The model under review builds one solid part; all positions refer to its coordinate system, in mm. Face numbers are marked on the shaded views. A direction names the side the tool comes from. Coordinates: 2 decimals unless noted, no trailing zeros. Write each loop counter-clockwise with the first axis right and the second up, starting at its lowest first coordinate (ties: lowest second). Pieces come first, ordered by that corner, then holes. Notation, with made-up numbers: (34.5, -28.75) - (46.5, -28.75) arc R10 cw to (46.5, -16.75) - close; hole circle Ø7 at (-24, -16). An arc over 180 degrees is marked (long way). Return JSON: item names as keys, results as strings. Group by question number.
(1) To check wall thickness, follow L1, parallel to X at y = -32, z = -29; L2, parallel to Z at x = -15, y = -6.5; L3, parallel to X at y = -39, z = -33.5. State the ranges of each line that lie inside material, in increasing order. Write a range as from..to.
(2) For pin 1 Ø3 at (x, y) = (18, -31.5) entering from +Z; pin 2 Ø12 at (x, y) = (-13, -12) entering from -Z; pin 3 Ø6 at (x, z) = (-10.5, -13.5) entering from +Y; pin 4 Ø1 at (y, z) = (-37.5, -35.5) entering from +X, all flat-tipped, find the tip position at first contact; note any pin that passes through.
(3) We need section C-C on z = -40. State the section outline as (x, y) points, then the cut area to 3 significant figures.
(4) We need section B-B on y = -6. State the section outline as (x, z) points.
(5) We need section D-D on x = 4.5. State the section outline as (y, z) points, then the cut area to 3 significant figures.
(6) Tool access review of the marked faces 1 and 2: name each direction out of +Z, -Z, +X, -X, +Y, -Y from which nothing blocks a thin tool from reaching the whole face with its end or side.
(7) We need section A-A on y = -21. State the section outline as (x, z) points, then the cut area to 3 significant figures.
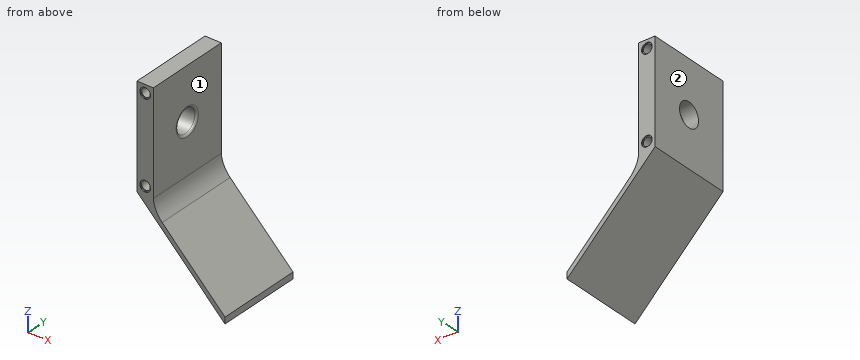
```python
from build123d import *

# Parameters (mm, degrees)
SKETCH1_W           = 25
SKETCH1_H           = 50
SKETCH1_R           = 3.4
BOSS_EXTRUDE1_DEPTH = 3
SKETCH2_W           = 50
SKETCH2_H           = 3
BOSS_EXTRUDE2_DEPTH = 8
SKETCH3_W           = 8
SKETCH3_H           = 50
BOSS_EXTRUDE3_DEPTH = 42
SKETCH4_R           = 2.65
CUT_EXTRUDE1_DEPTH  = 0.5
SKETCH5_R           = 5.888972746
CUT_EXTRUDE2_DEPTH  = 9
FILLET2_R           = 1
SKETCH6_R           = 12.6
BOSS_EXTRUDE4_DEPTH = 2
FILLET4_R           = 1
SKETCH8_R           = 1.589780168
SKETCH8_R_2         = 1.777428262
CUT_EXTRUDE3_DEPTH  = 10
SKETCH9_W           = 49.021678163
SKETCH9_H           = 20.976854622
CUT_EXTRUDE4_DEPTH  = 68.79439129
SKETCH11_R          = 2.1
CUT_EXTRUDE5_DEPTH  = 59.480168703
SKETCH14_R          = 2.6
CUT_EXTRUDE6_DEPTH  = 0.5
BOSS_EXTRUDE5_DEPTH = 42
FILLET5_R           = 15


with BuildPart() as part:
    # Sketch1 → Boss-Extrude1 (new body)
    with BuildSketch(Plane(origin=(0, 0, 0), x_dir=(1, 0, 0), z_dir=(0, 1, 0))):
        with Locations((2.276951673, 11.384758364)):
            Rectangle(SKETCH1_W, SKETCH1_H)
        with Locations(Location((1.276951673, 11.384758364, 0), (0, 0, 270))):
            Circle(SKETCH1_R, mode=Mode.SUBTRACT)
    extrude(amount=BOSS_EXTRUDE1_DEPTH)

    # Sketch2 → Boss-Extrude2 (add)
    with BuildSketch(Plane.ZY.offset(10.223048327)):
        with Locations((-11.384758364, 1.5)):
            Rectangle(SKETCH2_W, SKETCH2_H)
    extrude(amount=BOSS_EXTRUDE2_DEPTH)

    # Sketch3 → Boss-Extrude3 (add)
    with BuildSketch(Plane.XZ):
        with Locations((-14.223048327, -11.384758364)):
            Rectangle(SKETCH3_W, SKETCH3_H)
    extrude(amount=BOSS_EXTRUDE3_DEPTH)

    # Sketch4 → Cut-Extrude1 (cut)
    with BuildSketch(Plane(origin=(0, 3, 0), x_dir=(1, 0, 0), z_dir=(0, 1, 0))):
        with Locations(Location((-14.223048327, 32.384758364, 0), (0, 0, 270))):
            Circle(SKETCH4_R)
        with Locations(Location((-14.223048327, -9.615241636, 0), (0, 0, 270))):
            Circle(SKETCH4_R)
    cut_extrude1 = extrude(amount=-CUT_EXTRUDE1_DEPTH, mode=Mode.SUBTRACT)

    # Mirror1: Cut-Extrude1 across plane
    add(cut_extrude1.mirror(Plane.ZX.offset(-19.5)), mode=Mode.SUBTRACT)

    # Sketch5 → Cut-Extrude2 (cut)
    with BuildSketch(Plane.ZY.offset(18.223048327)):
        with Locations((-11.836279124, -21)):
            Circle(SKETCH5_R)
    extrude(amount=-CUT_EXTRUDE2_DEPTH, mode=Mode.SUBTRACT)

    # Fillet2
    fillet2_edges = [part.edges().sort_by_distance(p)[0] for p in [
        (-10.223048327, -21, -17.72525187),
    ]]
    fillet(fillet2_edges, radius=FILLET2_R)

    # Mirror2: Cut-Extrude1 across plane
    add(cut_extrude1.mirror(Plane.ZY.offset(1.723048327)), mode=Mode.SUBTRACT)

    # Sketch6 → Boss-Extrude4 (add)
    with BuildSketch(Plane(origin=(0, 3, 0), x_dir=(1, 0, 0), z_dir=(0, 1, 0))):
        with BuildLine():
            Line((14.776951673, 5.825082115), (14.776951673, 16.944434614))
            ThreePointArc((14.776951673, 16.944434614), (-13.323048327, 11.384758364), (14.776951673, 5.825082115))
        make_face()
        with Locations(Location((1.276951673, 11.384758364, 0), (0, 0, 270))):
            Circle(SKETCH6_R, mode=Mode.SUBTRACT)
    extrude(amount=BOSS_EXTRUDE4_DEPTH)

    # Fillet4
    # the kernel refuses this fillet: 1 mm, written as the material it takes off along each edge
    with BuildSketch(Plane(origin=(14.776951673, 5, -3.325082115), x_dir=(0, -1, 0), z_dir=(0, 0, -1))) as fillet4_piece_1:
        with BuildLine():
            CenterArc((FILLET4_R, FILLET4_R), FILLET4_R, 180, 90)
            Line((0, FILLET4_R), (0, 0))
            Line((0, 0), (FILLET4_R, 0))
        make_face()
    extrude(amount=16.119352499, mode=Mode.SUBTRACT)

    # Sketch8 → Cut-Extrude3 (cut)
    with BuildSketch(Plane(origin=(0, 3, 0), x_dir=(1, 0, 0), z_dir=(0, 1, 0))):
        with Locations(Location((1.276951673, 19.884758364, 0), (0, 0, 270))):
            Circle(SKETCH8_R)
        with Locations(Location((1.276951673, 2.884758364, 0), (0, 0, 270))):
            Circle(SKETCH8_R_2)
    extrude(amount=-CUT_EXTRUDE3_DEPTH, mode=Mode.SUBTRACT)

    # Sketch9 → Cut-Extrude4 (cut, through all)
    with BuildSketch(Plane.XY.offset(13.615241636)):
        with Locations((-9.733887409, 10.488427311)):
            Rectangle(SKETCH9_W, SKETCH9_H)
    extrude(amount=-CUT_EXTRUDE4_DEPTH, mode=Mode.SUBTRACT)

    # Sketch11 → Cut-Extrude5 (cut, through all)
    with BuildSketch(Plane(origin=(0, 0, 0), x_dir=(1, 0, 0), z_dir=(0, 1, 0))):
        with Locations(Location((-14.223048327, 32.384758364, 0), (0, 0, 270))):
            Circle(SKETCH11_R)
    cut_extrude5 = extrude(amount=-CUT_EXTRUDE5_DEPTH, mode=Mode.SUBTRACT)

    # Mirror3: Cut-Extrude5 across plane
    add(cut_extrude5.mirror(Plane.XY.offset(-11.384758364)), mode=Mode.SUBTRACT)

    # Sketch14 → Cut-Extrude6 (cut)
    with BuildSketch(Plane(origin=(0, 0, 0), x_dir=(1, 0, 0), z_dir=(0, 1, 0))):
        with Locations(Location((-14.223048327, -9.615241636, 0), (0, 0, 270))):
            Circle(SKETCH14_R)
    cut_extrude6 = extrude(amount=-CUT_EXTRUDE6_DEPTH, mode=Mode.SUBTRACT)

    # Mirror4: Cut-Extrude6 across plane
    add(cut_extrude6.mirror(Plane.XY.offset(-11.384758364)), mode=Mode.SUBTRACT)

    # Sketch15 → Boss-Extrude5 (add)
    with BuildSketch(Plane(origin=(0, 0, 0), x_dir=(1, 0, 0), z_dir=(0, 1, 0))):
        Polygon((-18.223048327, 36.384758364), (24.976951673, 79.584758364), (24.976951673, 76.472221629), (-15.110511592, 36.384758364), align=None)
    extrude(amount=-BOSS_EXTRUDE5_DEPTH)

    # Fillet5
    # the kernel refuses this fillet: 15 mm, written as the material it adds along each edge
    with BuildSketch(Plane(origin=(-15.110511592, 0, -36.384758364), x_dir=(1, 0, 0), z_dir=(0, -1, 0))) as fillet5_piece_1:
        with BuildLine():
            CenterArc((19.822892097, 1.390311339), FILLET5_R, 185.31823153, 39.68176847)
            Line((9.216290379, -9.216290379), (0, 0))
            Line((0, 0), (4.887463265, 0))
        make_face()
    extrude(amount=42)


solid = part.part
```
Ans:
{
 "1": {"L1": "-18.22..-10.22", "L2": "-39.61..-34.34, -30.43..7.66, 11.57..13.62", "L3": "-18.22..-16, -12.44..-10.22"},
 "2": {"pin 1": "z = -68", "pin 2": "z = -47.61", "pin 3": "y = 0", "pin 4": "x = -10.22"},
 "3": {"outline": "(-14.61, -42) - (-9.43, -42) - (-9.43, 0) - (-14.61, 0) - close", "area": "218 mm²"},
 "4": {"outline": "(-18.22, -36.38) - (24.98, -79.58) - (24.98, -76.47) - (-5.89, -45.6) arc R15 cw to (-10.22, -36.38) - (-10.22, 13.62) - (-18.22, 13.62) - close; hole circle Ø4.2 at (-14.22, -32.38); hole circle Ø4.2 at (-14.22, 9.62)"},
 "5": {"outline": "(-42, -59.11) - (0, -59.11) - (0, -56) - (-42, -56) - close", "area": "131 mm²"},
 "6": {"face 1": "+Z, +X, +Y, -Y", "face 2": "+Z, -Z, -X, +Y, -Y"},
 "7": {"outline": "(-18.22, -36.38) - (24.98, -79.58) - (24.98, -76.47) - (-5.89, -45.6) arc R15 cw to (-10.22, -36.38) - (-10.22, -18.73) arc R1 ccw to (-11.22, -17.73) - (-18.22, -17.73) - close; (-18.22, -5.95) - (-11.22, -5.95) arc R1 ccw to (-10.22, -4.95) - (-10.22, 13.62) - (-18.22, 13.62) - close; hole circle Ø4.2 at (-14.22, -32.38); hole circle Ø4.2 at (-14.22, 9.62)", "area": "424 mm²"}
}
